Read the model definition and answer for the solid it produces. Units are mm, in the model's axes. A direction names the side the tool comes from. Give positions to 0.01 mm unless a question says otherwise; leave off trailing zeros. Write each loop counter-clockwise with the first axis right and the second up, starting at its lowest first coordinate (ties: lowest second). Pieces come first, ordered by that corner, then holes. Notation, with made-up numbers: (39.25, 54) - (63.25, 54) arc R32 cw to (63.25, 87) - close; hole circle Ø1 at (16.25, 70.5). An arc over 180 degrees is marked (long way). Answer as a JSON object with one key per item and string values. Group by question number.
Solid Edge part; units mm, degrees
sketch "Sketch1" plane through (0, 0, 0) normal (0, 0, 1) x (1, 0, 0)
  line L0 (0, 3.5) -> (0, 2.6)
  line L1 (0, 2.6) -> (0.6, 2.6)
  line L2 (0.6, 2.6) -> (0.9077, 2.067)
  line L3 (0.9077, 2.067) -> (9.25, 2.067)
  line L4 (9.25, 2.067) -> (9.5, 2.5)
  line L5 (9.5, 2.5) -> (9.5, 2.86)
  line L6 (9.5, 2.86) -> (9.2, 3.16)
  line L7 (9.2, 3.16) -> (8.4, 3.16)
  line L8 (8.4, 3.16) -> (8.4, 2.935)
  line L9 (8.4, 2.935) -> (7.1, 2.935)
  line L10 (7.1, 2.935) -> (6.66, 3.375)
  line L11 (6.66, 3.375) -> (3.8, 3.375)
  line L12 (3.8, 3.375) -> (3.8, 3)
  line L13 (3.8, 3) -> (2.8, 3)
  line L14 (2.8, 3) -> (2.8, 3.5)
  line L15 (2.8, 3.5) -> (0, 3.5)
revolve "RevolvedProtrusion1" add sketch "Sketch1" angle 360 about axis through (9.5, 0, 0) along (-1, 0, 0)
cosmetic_thread "Thread1"
properties part number "KerbKonus 860000050800"
1) Flat-ended cylindrical pins translate along their axes: pin 1 Ø1.5 at (x, y) = (8, 1) entering from +Z; pin 2 Ø2 at (x, z) = (7, 2.5) entering from +Y; pin 3 Ø3.5 at (y, z) = (1, 1.5) entering from +X; pin 4 Ø1.5 at (x, z) = (6.5, 0.5) entering from -Y (3 decimals). Find the tip coordinate at first contact, or state that the pin passes through.
2) Find section D-D, the plane x = 3. Write down the section's boundary in (y, z).
3) Find section C-C, the plane x = 4.75. Write down the section's boundary in (y, z) (3 decimals).
4) Find the intervals of material crossed by line 1 (Y direction, x = 5.5, z = 0) (3 decimals); line 2 (Z direction, x = 0.1, y = 0), in increasing order. Write a range as [from, to].
5) Which of the six approach directions +Z, -Z, +X, -X, +Y, -Y give full straight-line access (tool end or side, diameter ignored) to faces 4 (the cylindrical face through (8.794, 1.699, -2.665)), 5 (the cylindrical face through (3, -3, 0)), 6 (the cylindrical face through (0.304, -0.338, 2.578)), 7 (the cylindrical face through (5.14, -1.64, -1.26))?
6) For a pull along X with two mould halves and no side action, classify faces 1 (the cylindrical face through (1.38, 3.233, 1.341)), 2 (the cylindrical face through (7.741, -2.163, -1.984)), 3 (the flat face through (0, 0, -3)) as released by +X, released by -X, zero draft, split by the parting line, or undercut.
Values follow:
{
 "1": {"pin 1": "stops at z = 3.14", "pin 2": "stops at y = 2.99", "pin 3": "stops at x = 9.5", "pin 4": "stops at y = -3.375"},
 "2": {"outline": "circle Ø6 at (0, 0); hole circle Ø4.13 at (0, 0)"},
 "3": {"outline": "circle Ø6.75 at (0, 0); hole circle Ø4.134 at (0, 0)"},
 "4": {"line 1": "y = [-3.375, -2.067], [2.067, 3.375]", "line 2": "z = [-3.5, -2.6], [2.6, 3.5]"},
 "5": {"face 4": "+X", "face 5": "none", "face 6": "-X", "face 7": "+X, -X"},
 "6": {"face 1": "zero draft", "face 2": "undercut", "face 3": "released by -X"}
}
